```python
from build123d import *

# Parameters (mm, degrees)
BOX_W           = 78
BOX_H           = 30
BOX_DEPTH       = 3
SKETCH001_W     = 20
SKETCH001_H     = 10
PAD_DEPTH       = 5
SKETCH002_W     = 16
SKETCH002_H     = 3
POCKET_DEPTH    = 20.001
POCKET001_DEPTH = 5
FILLET_R        = 1


with BuildPart() as part:
    # Box → Box (join)
    with BuildSketch(Plane.XY):
        with Locations((39, 15)):
            Rectangle(BOX_W, BOX_H)
    extrude(amount=BOX_DEPTH)

    # Sketch001 (on Face6 of Box) → Pad (join)
    with BuildSketch(Plane.XY.offset(3)):
        with Locations((39, 15)):
            Rectangle(SKETCH001_W, SKETCH001_H)
    extrude(amount=PAD_DEPTH)

    # Sketch002 (on Face8 of Pad) → Pocket (cut, through all)
    with BuildSketch(Plane.XZ.offset(-10)):
        with Locations((39, 4.501)):
            Rectangle(SKETCH002_W, SKETCH002_H)
    extrude(amount=-POCKET_DEPTH, mode=Mode.SUBTRACT)

    # Sketch003 (on Face11 of Pocket) → Pocket001 (cut)
    with BuildSketch(Plane.XY.offset(8)):
        with BuildLine():
            ThreePointArc((49, 10), (39, 14.142136), (29, 10))
            Line((29, 10), (49, 10))
        make_face()
    extrude(amount=-POCKET001_DEPTH, mode=Mode.SUBTRACT)

    # Fillet
    fillet_edges = [part.edges().sort_by_distance(p)[0] for p in [
        (49, 10, 5.5),
        (49, 20, 5.5),
        (29, 20, 5.5),
        (29, 10, 5.5),
    ]]
    fillet(fillet_edges, radius=FILLET_R)


solid = part.part
```
Model file for the job. Use its own axes, mm. A direction names the side the tool comes from. Round coordinates to 2 decimals unless told otherwise and drop trailing zeros. Write each loop counter-clockwise with the first axis right and the second up, starting at its lowest first coordinate (ties: lowest second). Pieces come first, ordered by that corner, then holes. Notation, with made-up numbers: (85.25, -10.5) -> (89.25, -10.5) arc R18 cw to (89.25, 3.5) -> close; hole circle Ø11 at (55, -10.75). An arc over 180 degrees is marked (long way). Answer as CSV lines item,"result".
1. Drill centre lines: line 1 (X direction, y = 18.5, z = 3.5); line 2 (Z direction, x = 35, y = 19); line 3 (Z direction, x = 24, y = 14.25). Where is each one in solid material? Low to high.
Resolved:
line 1,"29 to 31, 47 to 49"
line 2,"0 to 3, 6 to 8"
line 3,"0 to 3"
2. Slice it at C-C, the plane x = 60. List the corners of the cut face in (y, z), plus the area to 3 significant figures.
Resolved:
outline,"(0, 0) -> (30, 0) -> (30, 3) -> (0, 3) -> close"
area,"90.0 mm²"
3. Slice it at D-D, the plane y = 27.5. List the corners of the cut face in (x, z), plus the area to 3 significant figures.
Resolved:
outline,"(0, 0) -> (78, 0) -> (78, 3) -> (0, 3) -> close"
area,"234 mm²"
4. Slice it at B-B, the plane z = 5. List the corners of the cut face in (x, y).
Resolved:
outline,"(29, 12.18) arc R1 ccw to (30.59, 11.37) arc R14.14 cw to (31, 11.66) -> (31, 20) -> (30, 20) arc R1 ccw to (29, 19) -> close; (47, 11.66) arc R14.14 cw to (47.41, 11.37) arc R1 ccw to (49, 12.18) -> (49, 19) arc R1 ccw to (48, 20) -> (47, 20) -> close"
5. Tool access for faces 1 (the face through (39, 17, 6.001)), 2 (the face through (29, 16, 5)), 3 (the face through (29.54, 11.29, 5.54)): list every direction of +Z, -Z, +X, -X, +Y, -Y with a clear straight run to the whole face (end or side of a thin tool).
Resolved:
face 1,"+Y, -Y"
face 2,"+Z, -X, +Y, -Y"
face 3,"+Z, -Y"
6. Pin check, flat tips, straight feed: pin 1 Ø4 at (y, z) = (22.5, 6) entering from +X; pin 2 Ø4 at (x, z) = (37.5, 5.5) entering from +Y; pin 3 Ø2.5 at (y, z) = (18, 5) entering from +X. Stop position of each tip, or through.
Resolved:
pin 1,"through"
pin 2,"y = 20"
pin 3,"x = 49"
